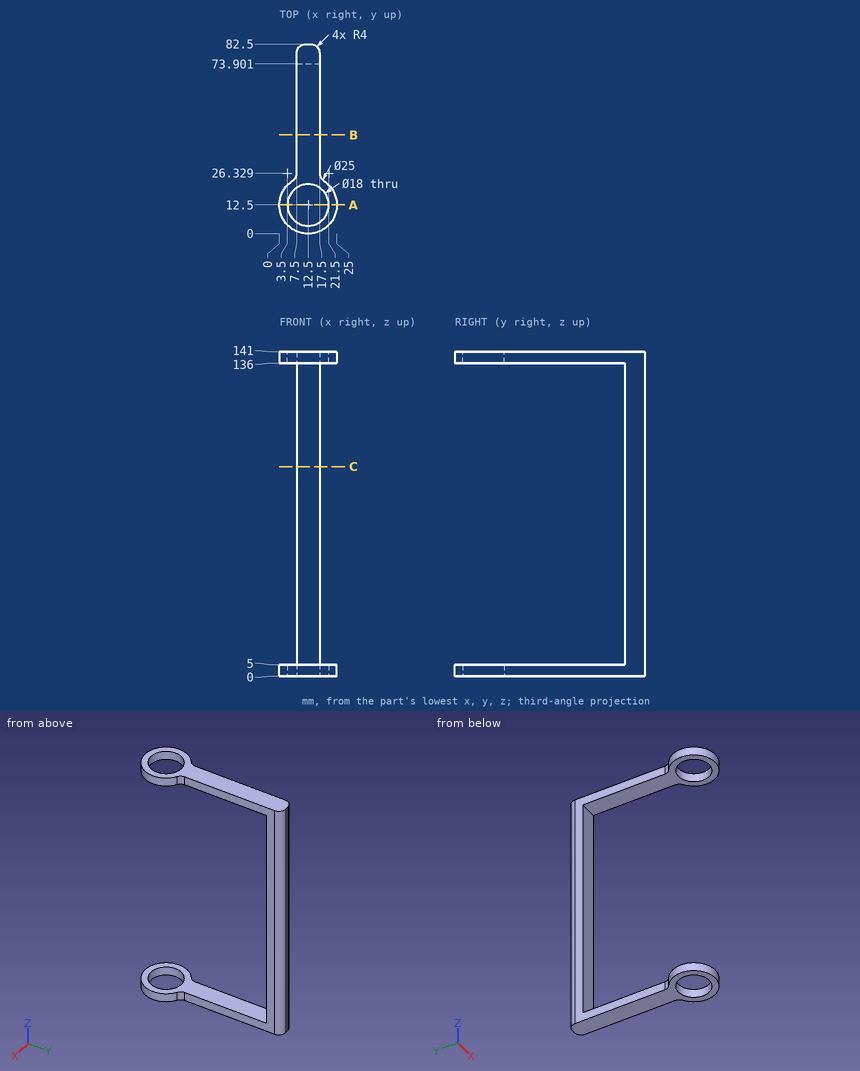
Source: three-view drawing plus pictorial views. Frame: mm from the lowest corner of the part. Round coordinates to 2 decimals unless told otherwise and drop trailing zeros. Order: outer loops, then holes, each group sorted by start corner. A loop starts at its lowest first (then second) coordinate and runs counter-clockwise, first axis right, second up. Notation, with made-up numbers: (-12, -14.5) -> (42, -14.5) arc R14 ccw to (42, -10.5) -> close; hole circle Ø11 at (19, 37.5). An arc over 180 degrees is marked (long way). Use CSV: the item, a comma, the result in double quotes. Start each with the question number.
1) Material intervals for line 1 along Z through (x, y) = (11, 37.5); line 2 along Y through (x, z) = (12.5, 139.8); line 3 along X through (y, z) = (77, 132), sorted ascending. Write a range as from..to.
2) Section A-A (y = 12.5). Return the cut outline in (x, z).
3) First-contact query: pin 1 Ø12 at (x, z) = (22, 115.5) entering from +Y; pin 2 Ø11 at (x, z) = (13.5, 52) entering from -Y. Flat tips, straight axial feed; report the tip coordinate or a pass-through.
4) Section B-B (y = 43). Return the cut outline in (x, z), and give its area (3 significant figures).
5) Section C-C (z = 91). Return the cut outline in (x, y), and give its area (3 significant figures).
Returned:
1,line 1,"z = 0..5, 136..141"
1,line 2,"y = 0..3.5, 21.5..82.5"
1,line 3,"x = 7.5..17.5"
2,outline,"(0, 0) -> (3.5, 0) -> (3.5, 5) -> (0, 5) -> close; (0, 136) -> (3.5, 136) -> (3.5, 141) -> (0, 141) -> close; (21.5, 0) -> (25, 0) -> (25, 5) -> (21.5, 5) -> close; (21.5, 136) -> (25, 136) -> (25, 141) -> (21.5, 141) -> close"
3,pin 1,"stops at y = 81.62"
3,pin 2,"stops at y = 73.9"
4,outline,"(7.5, 0) -> (17.5, 0) -> (17.5, 5) -> (7.5, 5) -> close; (7.5, 136) -> (17.5, 136) -> (17.5, 141) -> (7.5, 141) -> close"
4,area,"100 mm²"
5,outline,"(7.5, 73.9) -> (17.5, 73.9) -> (17.5, 78.5) arc R4 ccw to (13.5, 82.5) -> (11.5, 82.5) arc R4 ccw to (7.5, 78.5) -> close"
5,area,"79.1 mm²"
